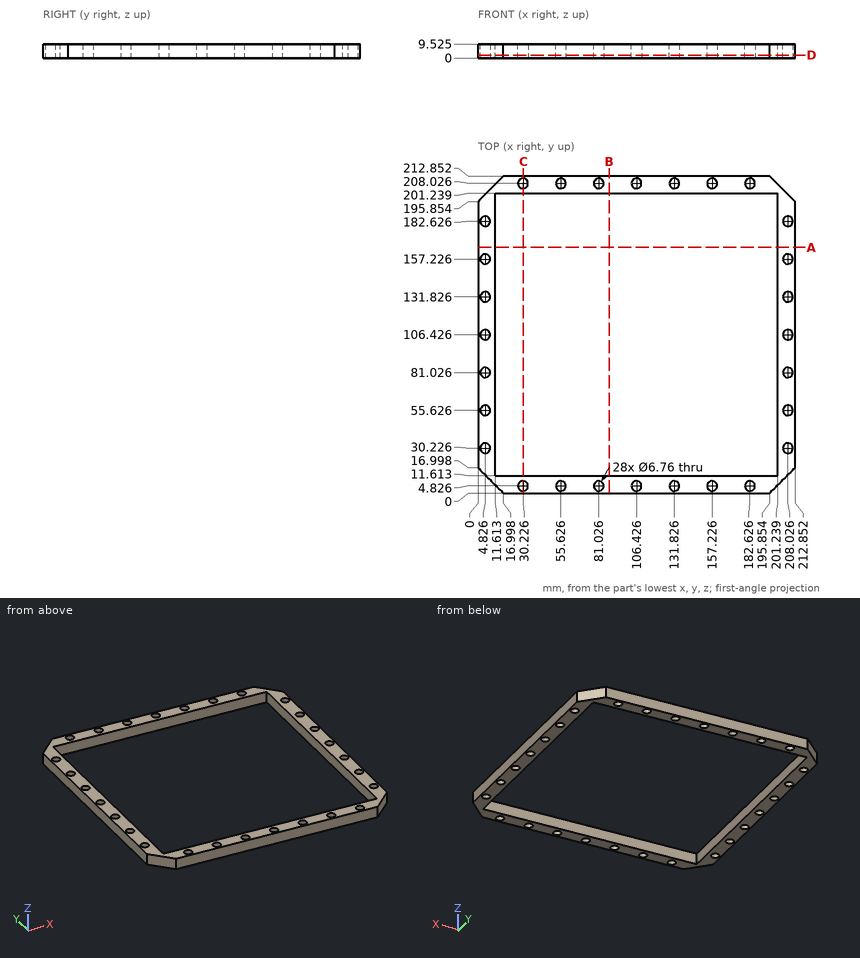
Part print with two shaded views. Sizes in mm from the minimum x, y, z corner. Give positions to 0.01 mm unless a question says otherwise; leave off trailing zeros. Order: outer loops, then holes, each group sorted by start corner. A loop starts at its lowest first (then second) coordinate and runs counter-clockwise, first axis right, second up. Notation, with made-up numbers: M -29,43 L 17,43 A25 cw 17,55 Z; hole C 23.25,39 d6. An arc over 180 degrees is marked long. Write item = value, one per line.
Q1. Cut at D-D, the plane z = 2. Count the separate pieces of the cut face and the enclosed holes in it.
Derived:
separate_pieces = 1
enclosed_holes = 29
Q2. Cut at C-C, the plane x = 30.5. List the corners of the cut face in (y, z) (1 decimal).
Derived:
outline = M 0,0 L 1.5,0 L 1.5,9.5 L 0,9.5 Z; M 8.2,0 L 11.6,0 L 11.6,9.5 L 8.2,9.5 Z; M 201.2,0 L 204.7,0 L 204.7,9.5 L 201.2,9.5 Z; M 211.4,0 L 212.9,0 L 212.9,9.5 L 211.4,9.5 Z
Q3. Cut at A-A, the plane y = 165. List the corners of the cut face in (x, z) (1 decimal), then the cut area to 3 significant figures.
Derived:
outline = M 0,0 L 11.6,0 L 11.6,9.5 L 0,9.5 Z; M 201.2,0 L 212.9,0 L 212.9,9.5 L 201.2,9.5 Z
area = 221 mm2
Q4. Drill centre lines: line 1 (Y direction, x = 132, z = 4.5); line 2 (Y direction, x = 81, z = 3.5). Where is each one in solid material? Low to high. Write a range as [from, to].
Derived:
line_1 = [0, 1.45], [8.2, 11.61], [201.24, 204.65], [211.4, 212.85]
line_2 = [0, 1.45], [8.21, 11.61], [201.24, 204.65], [211.41, 212.85]
